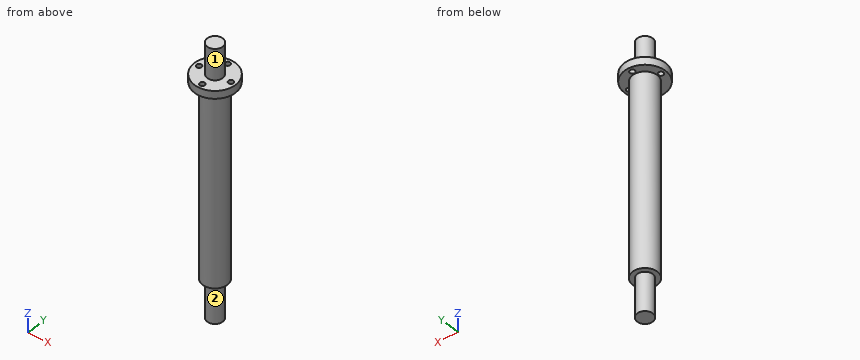
from build123d import *

# Parameters (mm, degrees)
SZKIC1_R                    = 26.376993093
SZKIC1_R_2                  = 3.228518126
DODANIE_WYCI_GNI_CIE1_DEPTH = 10
SZKIC2_R                    = 10
DODANIE_WYCI_GNI_CIE2_DEPTH = 40
SZKIC3_R                    = 15.88
DODANIE_WYCI_GNI_CIE3_DEPTH = 300
SZKIC4_R                    = 15.88
SZKIC4_R_2                  = 10
WYTNIJ_WYCI_GNI_CIE1_DEPTH  = 50


with BuildPart() as part:
    # Szkic1 → Dodanie-wyciągnięcie1 (new body)
    with BuildSketch(Plane.XY):
        Circle(SZKIC1_R)
        with Locations((0, 20)):
            Circle(SZKIC1_R_2, mode=Mode.SUBTRACT)
        with Locations((20, 0)):
            Circle(SZKIC1_R_2, mode=Mode.SUBTRACT)
        with Locations((0, -20)):
            Circle(SZKIC1_R_2, mode=Mode.SUBTRACT)
        with Locations((-20, 0)):
            Circle(SZKIC1_R_2, mode=Mode.SUBTRACT)
    extrude(amount=DODANIE_WYCI_GNI_CIE1_DEPTH)

    # Szkic2 → Dodanie-wyciągnięcie2 (add)
    with BuildSketch(Plane.XY.offset(10)):
        Circle(SZKIC2_R)
    extrude(amount=DODANIE_WYCI_GNI_CIE2_DEPTH)

    # Szkic3 → Dodanie-wyciągnięcie3 (add)
    with BuildSketch(Plane(origin=(0, 0, 0), x_dir=(-1, 0, 0), z_dir=(0, 0, -1))):
        Circle(SZKIC3_R)
    extrude(amount=DODANIE_WYCI_GNI_CIE3_DEPTH)

    # Szkic4 → Wytnij-wyciągnięcie1 (cut)
    with BuildSketch(Plane(origin=(0, 0, -300), x_dir=(-1, 0, 0), z_dir=(0, 0, -1))):
        Circle(SZKIC4_R)
        with Locations(Location((0, 0, 0), (0, 0, 180))):
            Circle(SZKIC4_R_2, mode=Mode.SUBTRACT)
    extrude(amount=-WYTNIJ_WYCI_GNI_CIE1_DEPTH, mode=Mode.SUBTRACT)


solid = part.part
Geometry check sheet. Reference: the model listing, model coordinates, mm. Face numbers are marked on the shaded views. A direction names the side the tool comes from. Round coordinates to 2 decimals unless told otherwise and drop trailing zeros. Write each loop counter-clockwise with the first axis right and the second up, starting at its lowest first coordinate (ties: lowest second). Pieces come first, ordered by that corner, then holes. Notation, with made-up numbers: (33, 57.5) -> (44, 57.5) arc R15 cw to (44, 77.5) -> close; hole circle Ø6 at (21, 18.25). An arc over 180 degrees is marked (long way). One line per item, written item: value. Start each with the question number.
(1) Cross-section at D-D, the plane z = -5.5. Record the cut outline in (x, y).
(2) Cross-section at A-A, the plane x = 0. Record the cut outline in (y, z).
(3) Access from +Z, -Z, +X, -X, +Y, -Y to the whole of each face (thin tool, end or side, straight path). Record for the marked faces 1 and 2.
(4) Go/stop test with flat-tipped pins: pin 1 Ø2 at (x, z) = (-8, -38) entering from +Y; pin 2 Ø10.5 at (x, y) = (-20, 0) entering from -Z; pin 3 Ø4 at (y, z) = (-3, -253) entering from +X. Record where each tip stops, or that it passes through.
(5) Cross-section at C-C, the plane y = 20. Record the cut outline in (x, z), and give its area (3 significant figures).
(6) Scan lines: line 1 (Y direction, x = 0, z = 2); line 2 (Z direction, x = -14.5, y = -19.5); line 3 (Y direction, x = 20, z = 2). Record each from-to range of solid material in increasing order. Write a range as [from, to].
Answer:
1. outline: circle Ø31.76 at (0, 0)
2. outline: (-26.38, 0) -> (-23.23, 0) -> (-23.23, 10) -> (-26.38, 10) -> close; (-16.77, 0) -> (-15.88, 0) -> (-15.88, -250) -> (-10, -250) -> (-10, -300) -> (10, -300) -> (10, -250) -> (15.88, -250) -> (15.88, 0) -> (16.77, 0) -> (16.77, 10) -> (10, 10) -> (10, 50) -> (-10, 50) -> (-10, 10) -> (-16.77, 10) -> close; (23.23, 0) -> (26.38, 0) -> (26.38, 10) -> (23.23, 10) -> close
3. face 1: +Z
3. face 2: -Z
4. pin 1: y = 14.25
4. pin 2: z = -250
4. pin 3: x = 9.95
5. outline: (-17.2, 0) -> (-3.23, 0) -> (-3.23, 10) -> (-17.2, 10) -> close; (3.23, 0) -> (17.2, 0) -> (17.2, 10) -> (3.23, 10) -> close
5. area: 279 mm²
6. line 1: [-26.38, -23.23], [-16.77, 16.77], [23.23, 26.38]
6. line 2: [0, 10]
6. line 3: [-17.2, -3.23], [3.23, 17.2]
